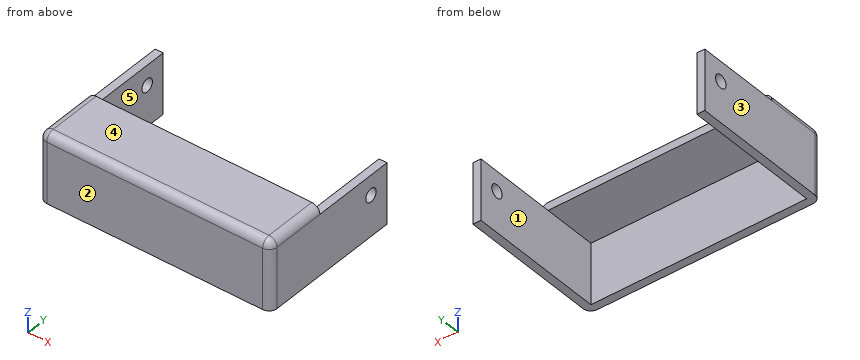
Autodesk Inventor part; units mm, degrees
ref_plane "YZ Plane" through (0, 0, 0) normal (1, 0, 0) x (0, 1, 0)
ref_plane "XZ Plane" through (0, 0, 0) normal (0, 1, 0) x (-1, 0, 0)
ref_plane "XY Plane" through (0, 0, 0) normal (0, 0, 1) x (1, 0, 0)
sketch "Sketch1" plane through (0, 0, 0) normal (0, 0, 1) x (1, 0, 0)
  line L0 (0, 0) -> (68.58, 0)
  line L1 (68.58, 0) -> (68.58, 17.018)
  line L2 (68.58, 17.018) -> (0, 17.018)
  line L3 (0, 17.018) -> (0, 0)
  dimension "d0" = 17.018
  dimension "d1" = 68.58
extrude "Extrusion1" add sketch "Sketch1" along normal blind 2.54
sketch "Sketch2" plane through (0, 0, 2.54) normal (0, 0, 1) x (1, 0, 0)
  line L0 (0, 0) -> (68.58, 0)
  line L1 (68.58, 0) -> (68.58, 17.018)
  line L2 (68.58, 17.018) -> (0, 17.018)
  line L3 (0, 17.018) -> (0, 0)
  line L4 (-2.54, 17.018) -> (71.12, 17.018)
  line L5 (71.12, 17.018) -> (71.12, -2.54)
  line L6 (71.12, -2.54) -> (-2.54, -2.54)
  line L7 (-2.54, -2.54) -> (-2.54, 17.018)
  dimension "d4" = 0
  dimension "d5" = 2.54
  dimension "d6" = 2.54
  dimension "d7" = 2.54
extrude "Extrusion2" add sketch "Sketch2" against normal blind 21.844 contours L0 L1 L4 L5 L6 L7 L3
fillet "Fillet1" radius 2.54 5 edges at (71.12, -2.54, -8.382) (-2.54, -2.54, -8.382) (34.29, -2.54, 2.54) (71.12, 7.239, 2.54) (-2.54, 7.239, 2.54)
sketch "Sketch3" plane through (0, 17.018, 0) normal (0, 1, 0) x (1, 0, 0)
  arc A0 (68.58, -2.54) -> (71.12, 0) centre (68.58, 0) ccw
  arc A1 (-2.54, 0) -> (0, -2.54) centre (0, 0) ccw
  line L0 (-2.54, 19.304) -> (0, 19.304)
  line L1 (0, 19.304) -> (0, 0)
  line L2 (0, 0) -> (-2.54, 0)
  line L3 (-2.54, 0) -> (-2.54, 19.304)
  line L4 (68.58, 0) -> (71.12, 0)
  line L5 (71.12, 0) -> (71.12, 19.304)
  line L6 (71.12, 19.304) -> (68.58, 19.304)
  line L7 (68.58, 19.304) -> (68.58, 0)
extrude "Extrusion3" add sketch "Sketch3" along normal blind 26.67
hole "Hole1" at (71.12, 37.338, -6.35) direction (-1, 0, 0) diameter 4.1656 end through all
equation "\"d6\" = d5"
equation "\"d7\" = d6"
properties part number "Back_Shield"
The model under review builds one solid part; all positions refer to its coordinate system, in mm. Face numbers are marked on the shaded views. A direction names the side the tool comes from. Give positions to 0.01 mm unless a question says otherwise; leave off trailing zeros. Write each loop counter-clockwise with the first axis right and the second up, starting at its lowest first coordinate (ties: lowest second). Pieces come first, ordered by that corner, then holes. Notation, with made-up numbers: (-7, 52) - (-1, 52) arc R17 cw to (-1, 78) - close; hole circle Ø5 at (-12.5, 58.5). An arc over 180 degrees is marked (long way). Answer in a Markdown table with one row per item. Add a question column.
1. We need section D-D on x = 8. Write out the cut boundary in (y, z), then the cut area to 3 significant figures.
2. Wall thickness on line 1 along X through (y, z) = (24, -1.25); line 2 along Z through (x, y) = (68, 12.5); line 3 along Y through (x, z) = (48, -5.5): over which ranges is each line inside the solid? List them lowest first. Write a range as [from, to].
3. Insertion check: P1, Ø6, axis at x = 23, z = -11.5, coming from the +Y side; P2, Ø2, axis at x = 70, y = 24.5, coming from the +Z side; P3, Ø3, axis at x = 19, z = 2, coming from the +Y side; P4, Ø5.5, axis at y = 37.338, z = -6.35, coming from the -X side. Each pin has a flat end and moves straight along its axis. Give the tip position at first contact, or say it passes through.
4. We need section C-C on y = 2.5. Write out the cut boundary in (x, z).
5. We need section A-A on y = 27. Write out the cut boundary in (x, z), then the cut area to 3 significant figures.
6. Draft analysis for pull direction X (two halves, no side actions). For the marked faces 3, 4 and 5, state which applies: +X half, -X half, draft (parallel to the pull), parting line (faces both ways), or undercut.
7. We need section B-B on z = -6.35. Write out the cut boundary in (x, y), then the cut area to 3 significant figures.
8. Tool access review of the marked faces 1 and 2: name each direction out of +Z, -Z, +X, -X, +Y, -Y from which nothing blocks a thin tool from reaching the whole face with its end or side.
Ans:
| question | item | result |
|---|---|---|
| 1 | outline | (-2.54, -19.3) - (0, -19.3) - (0, 0) - (17.02, 0) - (17.02, 2.54) - (0, 2.54) arc R2.54 ccw to (-2.54, 0) - close |
| 1 | area | 97.3 mm^2 |
| 2 | line 1 | x = [-2.54, 0], [68.58, 71.12] |
| 2 | line 2 | z = [0, 2.54] |
| 2 | line 3 | y = [-2.54, 0] |
| 3 | P1 | stops at y = 0 |
| 3 | P2 | stops at z = 0 |
| 3 | P3 | stops at y = 17.02 |
| 3 | P4 | stops at x = -2.54 |
| 4 | outline | (-2.54, -19.3) - (0, -19.3) - (0, 0) - (68.58, 0) - (68.58, -19.3) - (71.12, -19.3) - (71.12, 0) arc R2.54 ccw to (68.58, 2.54) - (0, 2.54) arc R2.54 ccw to (-2.54, 0) - close |
| 5 | outline | (-2.54, -19.3) - (0, -19.3) - (0, 0) - (-2.54, 0) - close; (68.58, -19.3) - (71.12, -19.3) - (71.12, 0) - (68.58, 0) - close |
| 5 | area | 98.1 mm^2 |
| 6 | face 3 | -X half |
| 6 | face 4 | draft |
| 6 | face 5 | undercut |
| 7 | outline | (-2.54, 0) arc R2.54 ccw to (0, -2.54) - (68.58, -2.54) arc R2.54 ccw to (71.12, 0) - (71.12, 35.26) - (68.58, 35.26) - (68.58, 0) - (0, 0) - (0, 35.26) - (-2.54, 35.26) - close; (-2.54, 39.42) - (0, 39.42) - (0, 43.69) - (-2.54, 43.69) - close; (68.58, 39.42) - (71.12, 39.42) - (71.12, 43.69) - (68.58, 43.69) - close |
| 7 | area | 385 mm^2 |
| 8 | face 1 | -Z, +Y |
| 8 | face 2 | +Z, -Z, +X, -X, -Y |
